from build123d import *

# Parameters (mm, degrees)
F0_R     = 12.7
F0_W     = 1.27
F0_H     = 1.27
F1_DEPTH = 38.1


with BuildPart() as f1:
    # F0 (on Top) → F1 (new body, symmetric)
    with BuildSketch(Plane.XY):
        Circle(F0_R)
        with BuildLine():
            Line((11.1125, 0.635), (11.1125, 0))
            Line((11.1125, 0), (11.1125, -0.635))
            Line((11.1125, -0.635), (11.0943423081, -0.635))
            ThreePointArc((11.0943423081, -0.635), (7.8577241059, -7.8577241059), (0.635, -11.0943423081))
            Line((0.635, -11.0943423081), (0.635, -11.1125))
            Line((0.635, -11.1125), (0, -11.1125))
            Line((0, -11.1125), (-0.635, -11.1125))
            Line((-0.635, -11.1125), (-0.635, -11.0943423081))
            ThreePointArc((-0.635, -11.0943423081), (-7.8577241059, -7.8577241059), (-11.0943423081, -0.635))
            Line((-11.0943423081, -0.635), (-11.1125, -0.635))
            Line((-11.1125, -0.635), (-11.1125, 0))
            Line((-11.1125, 0), (-11.1125, 0.635))
            Line((-11.1125, 0.635), (-11.0943423081, 0.635))
            ThreePointArc((-11.0943423081, 0.635), (-7.8577241059, 7.8577241059), (-0.635, 11.0943423081))
            Line((-0.635, 11.0943423081), (-0.635, 11.1125))
            Line((-0.635, 11.1125), (0, 11.1125))
            Line((0, 11.1125), (0.635, 11.1125))
            Line((0.635, 11.1125), (0.635, 11.0943423081))
            ThreePointArc((0.635, 11.0943423081), (7.8577241059, 7.8577241059), (11.0943423081, 0.635))
            Line((11.0943423081, 0.635), (11.1125, 0.635))
        make_face(mode=Mode.SUBTRACT)
        with BuildLine():
            Line((-0.635, -0.635), (-0.635, 0.635))
            Line((-0.635, 0.635), (-11.0943423081, 0.635))
            ThreePointArc((-11.0943423081, 0.635), (-11.1079596495, 0.3176297773), (-11.1125, 0))
            ThreePointArc((-11.1125, 0), (-11.1079596495, -0.3176297773), (-11.0943423081, -0.635))
            Line((-11.0943423081, -0.635), (-0.635, -0.635))
        make_face()
        with BuildLine():
            Line((0.635, 0.635), (0.635, 11.0943423081))
            ThreePointArc((0.635, 11.0943423081), (0.3176297773, 11.1079596495), (0, 11.1125))
            ThreePointArc((0, 11.1125), (-0.3176297773, 11.1079596495), (-0.635, 11.0943423081))
            Line((-0.635, 11.0943423081), (-0.635, 0.635))
            Line((-0.635, 0.635), (0.635, 0.635))
        make_face()
        with BuildLine():
            ThreePointArc((0, -11.1125), (0.3176297773, -11.1079596495), (0.635, -11.0943423081))
            Line((0.635, -11.0943423081), (0.635, -0.635))
            Line((0.635, -0.635), (-0.635, -0.635))
            Line((-0.635, -0.635), (-0.635, -11.0943423081))
            ThreePointArc((-0.635, -11.0943423081), (-0.3176297773, -11.1079596495), (0, -11.1125))
        make_face()
        with BuildLine():
            ThreePointArc((11.0943423081, -0.635), (11.1079596495, -0.3176297773), (11.1125, 0))
            ThreePointArc((11.1125, 0), (11.1079596495, 0.3176297773), (11.0943423081, 0.635))
            Line((11.0943423081, 0.635), (0.635, 0.635))
            Line((0.635, 0.635), (0.635, -0.635))
            Line((0.635, -0.635), (11.0943423081, -0.635))
        make_face()
        Rectangle(F0_W, F0_H)
        with BuildLine():
            ThreePointArc((-0.635, 11.0943423081), (-0.3176297773, 11.1079596495), (0, 11.1125))
            Line((0, 11.1125), (-0.635, 11.1125))
            Line((-0.635, 11.1125), (-0.635, 11.0943423081))
        make_face()
        with BuildLine():
            ThreePointArc((0, 11.1125), (0.3176297773, 11.1079596495), (0.635, 11.0943423081))
            Line((0.635, 11.0943423081), (0.635, 11.1125))
            Line((0.635, 11.1125), (0, 11.1125))
        make_face()
        with BuildLine():
            ThreePointArc((-11.1125, 0), (-11.1079596495, 0.3176297773), (-11.0943423081, 0.635))
            Line((-11.0943423081, 0.635), (-11.1125, 0.635))
            Line((-11.1125, 0.635), (-11.1125, 0))
        make_face()
        with BuildLine():
            Line((-11.1125, -0.635), (-11.0943423081, -0.635))
            ThreePointArc((-11.0943423081, -0.635), (-11.1079596495, -0.3176297773), (-11.1125, 0))
            Line((-11.1125, 0), (-11.1125, -0.635))
        make_face()
        with BuildLine():
            Line((11.1125, -0.635), (11.1125, 0))
            ThreePointArc((11.1125, 0), (11.1079596495, -0.3176297773), (11.0943423081, -0.635))
            Line((11.0943423081, -0.635), (11.1125, -0.635))
        make_face()
        with BuildLine():
            ThreePointArc((11.0943423081, 0.635), (11.1079596495, 0.3176297773), (11.1125, 0))
            Line((11.1125, 0), (11.1125, 0.635))
            Line((11.1125, 0.635), (11.0943423081, 0.635))
        make_face()
        with BuildLine():
            Line((0.635, -11.1125), (0.635, -11.0943423081))
            ThreePointArc((0.635, -11.0943423081), (0.3176297773, -11.1079596495), (0, -11.1125))
            Line((0, -11.1125), (0.635, -11.1125))
        make_face()
        with BuildLine():
            Line((-0.635, -11.1125), (0, -11.1125))
            ThreePointArc((0, -11.1125), (-0.3176297773, -11.1079596495), (-0.635, -11.0943423081))
            Line((-0.635, -11.0943423081), (-0.635, -11.1125))
        make_face()
    extrude(amount=F1_DEPTH, both=True)


solid = f1.part
The listing builds one solid part. Answer for the finished solid, in the listing's coordinates (mm). A direction names the side the tool comes from. Coordinates: 2 decimals unless noted, no trailing zeros. Write each loop counter-clockwise with the first axis right and the second up, starting at its lowest first coordinate (ties: lowest second). Pieces come first, ordered by that corner, then holes. Notation, with made-up numbers: M 66,87.25 L 119,87.25 A5 ccw 119,93.25 Z; hole C -11.75,43 d9. An arc over 180 degrees is marked long. Use one line per item in the form item = value.
Item 1: Given P1, Ø6, axis at x = 7.5, z = 5.5, coming from the -Y side; P2, Ø1, axis at y = -8.5, z = -22, coming from the -X side; P3, Ø11.5, axis at x = 7.5, z = 10, coming from the -Y side; P4, Ø10, axis at x = 1, z = -15, coming from the -Y side, each flat-ended and moving along its own axis, determine where each tip first touches the part or whether it passes through.
Model answer:
P1 = -11.88
P2 = -9.86
P3 = -12.58
P4 = -12.7
Item 2: Find section C-C, the plane x = 2.75. Give the vertices of the cut face in (y, z) (3 decimals), plus the area to 3 significant figures.
Model answer:
outline = M -12.399,-38.1 L -10.767,-38.1 L -10.767,38.1 L -12.399,38.1 Z; M -0.635,-38.1 L 0.635,-38.1 L 0.635,38.1 L -0.635,38.1 Z; M 10.767,-38.1 L 12.399,-38.1 L 12.399,38.1 L 10.767,38.1 Z
area = 345 mm2
Item 3: Find section A-A, the plane z = 17. Give the vertices of the cut face in (x, y) (1 decimal).
Model answer:
outline = C 0,0 d25.4; hole M -11.1,-0.6 A11.1 ccw -0.6,-11.1 L -0.6,-0.6 Z; hole M -11.1,0.6 L -0.6,0.6 L -0.6,11.1 A11.1 ccw Z; hole M 0.6,-11.1 A11.1 ccw 11.1,-0.6 L 0.6,-0.6 Z; hole M 0.6,0.6 L 11.1,0.6 A11.1 ccw 0.6,11.1 Z
Item 4: Find section B-B, the plane y = 3.5. Give the vertices of the cut face in (x, z) (3 decimals), plus the area to 3 significant figures.
Model answer:
outline = M -12.208,-38.1 L -10.547,-38.1 L -10.547,38.1 L -12.208,38.1 Z; M -0.635,-38.1 L 0.635,-38.1 L 0.635,38.1 L -0.635,38.1 Z; M 10.547,-38.1 L 12.208,-38.1 L 12.208,38.1 L 10.547,38.1 Z
area = 350 mm2
Item 5: For faces 4 (the face through (7.937, -7.777, 0.533)), 5 (the face through (0, 0, 38.1)), determine the directions among +Z, -Z, +X, -X, +Y, -Y from which every point of the face is accessible in a straight line to the end or side of a thin tool.
Model answer:
face_4 = +Z, -Z
face_5 = +Z, +X, -X, +Y, -Y
Item 6: The mould has two halves that part along Y. Classify faces 1 (the face through (0, 0, -38.1)), 2 (the face through (-2.75, -12.4, 0.53)), 3 (the face through (-0.635, -6, 1)): released by +Y, released by -Y, zero draft, split by the parting line, or undercut.
Model answer:
face_1 = zero draft
face_2 = split by the parting line
face_3 = undercut
Item 7: Find the intervals of material crossed by probe 1 along X at (y, z) = (-1, 0) (3 decimals); probe 2 along Y at (x, z) = (6, -32.5) (3 decimals); probe 3 along X at (y, z) = (5.25, -7) (3 decimals), in increasing order.
Model answer:
probe_1 = -12.661 to -11.067, -0.635 to 0.635, 11.067 to 12.661
probe_2 = -11.193 to -9.353, -0.635 to 0.635, 9.353 to 11.193
probe_3 = -11.564 to -9.794, -0.635 to 0.635, 9.794 to 11.564
